Autodesk Inventor part; units mm, degrees
ref_plane "YZ Plane" through (0, 0, 0) normal (1, 0, 0) x (0, 1, 0)
ref_plane "XZ Plane" through (0, 0, 0) normal (0, 1, 0) x (-1, 0, 0)
ref_plane "XY Plane" through (0, 0, 0) normal (0, 0, 1) x (1, 0, 0)
sketch "Sketch1" plane through (0, 0, 0) normal (0, 1, 0) x (-1, 0, 0)
  circle A0 centre (0, 0) radius 15.5
  dimension "d0" = 31
extrude "Extrusion1" add sketch "Sketch1" along normal blind 15
sketch "Sketch2" plane through (0, 0, 0) normal (0, -1, 0) x (1, 0, 0)
  circle A0 centre (0, 0) radius 14.2
  dimension "d3" = 28.4
extrude "Extrusion2" cut sketch "Sketch2" against normal blind 11
sketch "Sketch4" plane through (0, 11, 0) normal (0, -1, 0) x (1, 0, 0)
  point P0 (0, 0)
hole "Hole1" at (0, 11, 0) direction (0, 1, 0) diameter 4 depth 4 tip angle 118
properties part number "_3DPrint"
Input: part model. Units: mm. Frame: model coordinates. A direction names the side the tool comes from. Give positions to 0.01 mm unless a question says otherwise; leave off trailing zeros. Loops run counter-clockwise (first coordinate to the right, second up) from the corner with the lowest first, then second, coordinate; pieces in that order, holes last. Notation, with made-up numbers: (35.5, 44) -> (41.5, 44) arc R10 ccw to (41.5, 49) -> close; hole circle Ø11 at (10.25, 88.25). An arc over 180 degrees is marked (long way). Use a Markdown table: item, result.
Q1. Section query B-B, the plane x = 0. Return the cut outline in (y, z), plus the area to 3 significant figures.
Entries:
| item | result |
|---|---|
| outline | (0, -15.5) -> (15, -15.5) -> (15, -2) -> (11, -2) -> (11, -14.2) -> (0, -14.2) -> close; (0, 14.2) -> (11, 14.2) -> (11, 2) -> (15, 2) -> (15, 15.5) -> (0, 15.5) -> close |
| area | 137 mm² |
Q2. Section query A-A, the plane z = 0. Return the cut outline in (x, y), plus the area to 3 significant figures.
Entries:
| item | result |
|---|---|
| outline | (-15.5, 0) -> (-14.2, 0) -> (-14.2, 11) -> (-2, 11) -> (-2, 15) -> (-15.5, 15) -> close; (2, 11) -> (14.2, 11) -> (14.2, 0) -> (15.5, 0) -> (15.5, 15) -> (2, 15) -> close |
| area | 137 mm² |
Q3. Access query for faces 1 (the cylindrical face through (-1.85, 5.42, 14.08)), 2 (the flat face through (0, 15, -3)). Directions: +Z, -Z, +X, -X, +Y, -Y. A direction counts if a zero-diameter tool reaches every point of the face in a straight line with its end or side. Return the directions, or none.
Entries:
| item | result |
|---|---|
| face 1 | -Y |
| face 2 | +Z, -Z, +X, -X, +Y |
Q4. Section query C-C, the plane x = 12. Return the cut outline in (y, z).
Entries:
| item | result |
|---|---|
| outline | (0, -9.81) -> (15, -9.81) -> (15, 9.81) -> (0, 9.81) -> (0, 7.59) -> (11, 7.59) -> (11, -7.59) -> (0, -7.59) -> close |
Q5. Ray query, probe 1 along Z at (x, y) = (0, 5); probe 2 along Z at (x, y) = (0, 13.5); probe 3 along Y at (x, z) = (-7, -1). Return the intervals inside material, ascending. Write a range as from..to.
Entries:
| item | result |
|---|---|
| probe 1 | z = -15.5..-14.2, 14.2..15.5 |
| probe 2 | z = -15.5..-2, 2..15.5 |
| probe 3 | y = 11..15 |
Q6. First-contact query: P1, Ø1, axis at y = 2.5, z = 4.5, coming from the -X side (3 decimals); P2, Ø5, axis at x = 9, y = 10, coming from the -Z side; P3, Ø2, axis at x = 7, z = 0, coming from the -Y side; P4, Ø3, axis at x = -8.5, z = -11, coming from the -Y side. Flat tips, straight axial feed; report the tip coordinate or a pass-through.
Entries:
| item | result |
|---|---|
| P1 | stops at x = -14.975 |
| P2 | stops at z = -14.07 |
| P3 | stops at y = 11 |
| P4 | stops at y = 0 |
Q7. Section query D-D, the plane y = 2.5. Return the cut outline in (x, z), plus the area to 3 significant figures.
Entries:
| item | result |
|---|---|
| outline | circle Ø31 at (0, 0); hole circle Ø28.4 at (0, 0) |
| area | 121 mm² |
Q8. Pull-direction query (Z, two-part tool) for faces 3 (the cylindrical face through (2, 13, 0)), 4 (the cylindrical face through (2.018, 7.395, -15.368)), 5 (the flat face through (-7, 0, -13)); classes: pulls with the +Z half, pulls with the -Z half, needs draft (parallel to the pull), parting line crosses it, or undercut.
Entries:
| item | result |
|---|---|
| face 3 | undercut |
| face 4 | parting line crosses it |
| face 5 | needs draft |
